Here's how the part is built. I have some questions about the finished solid (model axes, mm). A direction names the side the tool comes from. Give positions to 0.01 mm unless a question says otherwise; leave off trailing zeros. Loops run counter-clockwise (first coordinate to the right, second up) from the corner with the lowest first, then second, coordinate; pieces in that order, holes last. Notation, with made-up numbers: (-22, 43) -> (28, 43) arc R18 ccw to (28, 77) -> close; hole circle Ø7 at (67, 38). An arc over 180 degrees is marked (long way). Answer in a Markdown table with one row per item. Add a question column.
Item 1: If we section it at A-A (z = -20): Write out the boundary of the cut face in (x, y).
Item 2: If we section it at B-B (y = 7): Write out the boundary of the cut face in (x, z), then the cut area to 3 significant figures.
Item 3: Which directions (+Z, -Z, +X, -X, +Y, -Y) give clear straight access to the entire face, cutting with the end or side of a thin tool? Please do faces 4 (the face through (0, 5.5, -24)), 5 (the face through (-14, 6, -24)), 6 (the face through (14, 6, -24)), 7 (the face through (13, 7, -11)), 8 (the face through (0, 6.5, -24)).
Item 4: For P1, Ø0.8, axis at x = -5.5, y = 6, coming from the -Z side; P2, Ø0.8, axis at y = 6, z = -20, coming from the -X side, each with a flat end and sliding along its axis, tell me the tip position at first contact or that it passes through.
Item 5: If we section it at D-D (z = -25): Write out the boundary of the cut face in (x, y).
Item 6: If we section it at C-C (x = -10): Write out the boundary of the cut face in (y, z).
Item 7: We'd pull the mould along Z, two halves only. Please class faces 1 (the face through (0, 7, -30)), 2 (the face through (-17, 7, -5)), 3 (the face through (0, 6.5, -33)): released by +Z, released by -Z, zero draft, split by the parting line, or undercut.
Item 8: If I drill on line 1 (Z direction, x = 10, y = 6.25); line 2 (Z direction, x = -4.5, y = 6.6); line 3 (Y direction, x = 4.5, z = -32.5), over which ranges is the centre line in solid material (lowest first)?
```python
from build123d import *

# Parameters (mm, degrees)
PAD113_DEPTH    = 2
SKETCH171_W     = 24
SKETCH171_H     = 12
POCKET010_DEPTH = 1
SKETCH172_W     = 46.237046
SKETCH172_H     = 37.182623
SKETCH172_W_2   = 28
SKETCH172_H_2   = 16
POCKET011_DEPTH = 1
SKETCH301_R     = 1.1
POCKET046_DEPTH = 5


with BuildPart() as part:
    # Sketch170 → Pad113 (new body)
    with BuildSketch(Plane.XZ):
        Polygon((21, -5), (21, -38.5), (-21, -38.5), (-21, -5), (-13, -5), (-13, -16), (13, -16), (13, -5), align=None)
    extrude(amount=PAD113_DEPTH)

    # Sketch171 (on Face9 of Pad113) → Pocket010 (cut)
    with BuildSketch(Plane(origin=(0, 0, 0), x_dir=(1, 0, 0), z_dir=(0, 1, 0))):
        with Locations((0, 24)):
            Rectangle(SKETCH171_W, SKETCH171_H)
    extrude(amount=-POCKET010_DEPTH, mode=Mode.SUBTRACT)

    # Sketch172 (on Face5 of Pocket010) → Pocket011 (cut)
    with BuildSketch(Plane.XZ.offset(2)):
        with Locations((0, -21.400319)):
            Rectangle(SKETCH172_W, SKETCH172_H)
        with Locations((0, -24)):
            Rectangle(SKETCH172_W_2, SKETCH172_H_2, mode=Mode.SUBTRACT)
    extrude(amount=-POCKET011_DEPTH, mode=Mode.SUBTRACT)

    # Sketch301 (on Face22 of Pocket011) → Pocket046 (cut)
    with BuildSketch(Plane.XZ.offset(2)):
        with Locations((10, -28)):
            Circle(SKETCH301_R)
        with Locations((-10, -20)):
            Circle(SKETCH301_R)
    extrude(amount=-POCKET046_DEPTH, mode=Mode.SUBTRACT)


with BuildPart() as part_1:
    # Body013 placement: moved
    add(part.part.moved(Location((0, 7.5, 0))))


solid = part_1.part
```
Recorded:
| question | item | result |
|---|---|---|
| 1 | outline | (-21, 6.5) -> (-14, 6.5) -> (-14, 5.5) -> (-11.1, 5.5) -> (-11.1, 6.5) -> (-12, 6.5) -> (-12, 7.5) -> (-21, 7.5) -> close; (-8.9, 5.5) -> (14, 5.5) -> (14, 6.5) -> (21, 6.5) -> (21, 7.5) -> (12, 7.5) -> (12, 6.5) -> (-8.9, 6.5) -> close |
| 2 | outline | (-21, -38.5) -> (21, -38.5) -> (21, -5) -> (13, -5) -> (13, -16) -> (-13, -16) -> (-13, -5) -> (-21, -5) -> close; hole (-12, -30) -> (12, -30) -> (12, -18) -> (-12, -18) -> close |
| 2 | area | 833 mm^2 |
| 3 | face 4 | +Z, -Z, +X, -X, -Y |
| 3 | face 5 | +Z, -Z, -X, -Y |
| 3 | face 6 | +Z, -Z, +X, -Y |
| 3 | face 7 | +Z, +Y, -Y |
| 3 | face 8 | +Y |
| 4 | P1 | stops at z = -32 |
| 4 | P2 | stops at x = -14 |
| 5 | outline | (-21, 6.5) -> (-14, 6.5) -> (-14, 5.5) -> (14, 5.5) -> (14, 6.5) -> (21, 6.5) -> (21, 7.5) -> (12, 7.5) -> (12, 6.5) -> (-12, 6.5) -> (-12, 7.5) -> (-21, 7.5) -> close |
| 6 | outline | (5.5, -32) -> (6.5, -32) -> (6.5, -38.5) -> (7.5, -38.5) -> (7.5, -30) -> (6.5, -30) -> (6.5, -21.1) -> (5.5, -21.1) -> close; (5.5, -18.9) -> (6.5, -18.9) -> (6.5, -18) -> (7.5, -18) -> (7.5, -16) -> (5.5, -16) -> close |
| 7 | face 1 | undercut |
| 7 | face 2 | released by +Z |
| 7 | face 3 | zero draft |
| 8 | line 1 | z = -32 to -29.1, -26.9 to -16 |
| 8 | line 2 | z = -38.5 to -30, -18 to -16 |
| 8 | line 3 | y = 6.5 to 7.5 |
